from build123d import *

# Parameters (mm, degrees)
F0_W     = 92.1698585153
F0_H     = 105.9397310019
F1_DEPTH = 25.4
F2_R     = 22.4003702497
F3_DEPTH = 25.4
F4_DEPTH = 25.4
F5_W     = 26.5126917511
F5_H     = 7.429022342
F6_DEPTH = 117.5708585153


with BuildPart() as f1:
    # F0 (on Top) → F1 (new body)
    with BuildSketch(Plane.XY):
        Rectangle(F0_W, F0_H)
    extrude(amount=F1_DEPTH)

    # F2 (on face) → F3 (join)
    with BuildSketch(Plane.XY.offset(25.4)):
        Circle(F2_R)
    extrude(amount=F3_DEPTH)

    # F4 (add): a face of the model
    f4_faces = [f1.faces().sort_by_distance(p)[0] for p in [
        (46.0849292576, 0, 12.7),
    ]]
    extrude(f4_faces, amount=F4_DEPTH)

    # F5 (on face) → F6 (cut, through all)
    with BuildSketch(Plane.YZ.offset(71.4849292576)):
        with Locations((-27.0254462957, 16.5118221194)):
            Rectangle(F5_W, F5_H)
    extrude(amount=-F6_DEPTH, mode=Mode.SUBTRACT)


solid = f1.part
For this review, take the finished solid that the model builds, in its own axes (mm). A direction names the side the tool comes from. Coordinates: 2 decimals unless noted, no trailing zeros. Loops run counter-clockwise (first coordinate to the right, second up) from the corner with the lowest first, then second, coordinate; pieces in that order, holes last. Notation, with made-up numbers: (47, -11) - (68, -11) arc R37 cw to (68, 27) - close; hole circle Ø5 at (-26.5, 54). An arc over 180 degrees is marked (long way). Return JSON: item names as keys, results as strings.
Item 1: Insertion check: pin 1 (10 mm diameter, centred on x = 32, y = -9.5, fed in from +Z); pin 2 (12 mm diameter, centred on x = -21, z = 29, fed in from -Y); pin 3 (1.5 mm diameter, centred on x = 20.5, z = 27, fed in from -Y). Each pin has a flat end and moves straight along its axis. Give the tip position at first contact, or say it passes through.
Determined:
{"pin 1": "stops at z = 25.4", "pin 2": "stops at y = -52.97", "pin 3": "stops at y = -10.57"}
Item 2: Mouldability with a two-part tool opening along Y and no side actions: class faces 4 (the flat face through (0, 0, 50.8)), 5 (the flat face through (12, 52.97, 13)), 6 (the flat face through (14, -40.282, 16)) as pulls with the +Y half, pulls with the -Y half, needs draft (parallel to the pull), parting line crosses it, or undercut.
Determined:
{"face 4": "needs draft", "face 5": "pulls with the +Y half", "face 6": "undercut"}
Item 3: For line 1 (Z direction, x = 46, y = -26.5); line 2 (Y direction, x = 17, z = 20); line 3 (Z direction, x = 10, y = 38), list the stretches that pass through material, from the lowest coordinate up.
Determined:
{"line 1": "z = 0 to 12.8, 20.23 to 25.4", "line 2": "y = -52.97 to -40.28, -13.77 to 52.97", "line 3": "z = 0 to 25.4"}
Item 4: Take a section at B-B (y = -35). Give the boundary of the cut face in (x, z), then the cut area to 3 significant figures.
Determined:
{"outline": "(-46.08, 0) - (71.48, 0) - (71.48, 12.8) - (-46.08, 12.8) - close; (-46.08, 20.23) - (71.48, 20.23) - (71.48, 25.4) - (-46.08, 25.4) - close", "area": "2,110 mm2"}
Item 5: Take a section at D-D (y = 0). Give the boundary of the cut face in (x, z), then the cut area to 3 significant figures.
Determined:
{"outline": "(-46.08, 0) - (71.48, 0) - (71.48, 25.4) - (22.4, 25.4) - (22.4, 50.8) - (-22.4, 50.8) - (-22.4, 25.4) - (-46.08, 25.4) - close", "area": "4,120 mm2"}
Item 6: Take a section at C-C (z = 18). Give the boundary of the cut face in (x, y), then the cut area to 3 significant figures.
Determined:
{"outline": "(-46.08, -52.97) - (71.48, -52.97) - (71.48, -40.28) - (-46.08, -40.28) - close; (-46.08, -13.77) - (71.48, -13.77) - (71.48, 52.97) - (-46.08, 52.97) - close", "area": "9,340 mm2"}
Item 7: For faces 1 (the flat face through (71.485, -1, 13)), 2 (the cylindrical face through (-4.856, -21.868, 37.922)), 3 (the flat face through (14, -27, 20.226)), list the 3-axis set-ups (+Z, -Z, +X, -X, +Y, -Y) from which the entire face can be reached by the end or side of a thin tool; tool diameter is ignored.
Determined:
{"face 1": "+Z, -Z, +X, +Y, -Y", "face 2": "+Z", "face 3": "+X, -X"}
Item 8: Take a section at A-A (x = 43.5). Give the boundary of the cut face in (y, z), then the cut area to 3 significant figures.
Determined:
{"outline": "(-52.97, 0) - (52.97, 0) - (52.97, 25.4) - (-52.97, 25.4) - close; hole (-40.28, 12.8) - (-13.77, 12.8) - (-13.77, 20.23) - (-40.28, 20.23) - close", "area": "2,490 mm2"}
